Autodesk Inventor part; units mm, degrees
ref_plane "YZ Plane" through (0, 0, 0) normal (1, 0, 0) x (0, 1, 0)
ref_plane "XZ Plane" through (0, 0, 0) normal (0, 1, 0) x (-1, 0, 0)
ref_plane "XY Plane" through (0, 0, 0) normal (0, 0, 1) x (1, 0, 0)
sketch "Эскиз1" plane through (0, 0, 0) normal (1, 0, 0) x (0, 1, 0)
  circle A0 centre (0, 0) radius 30.5
  dimension "d0" = 61
extrude "Выдавливание1" add sketch "Эскиз1" along normal blind 25
sketch "Эскиз2" plane through (25, 0, 0) normal (1, 0, 0) x (0, 0, -1)
  circle A0 centre (0, 0) radius 41
  dimension "d3" = 82
extrude "Выдавливание2" add sketch "Эскиз2" along normal blind 26
sketch "Эскиз3" plane through (0, 0, 0) normal (0, 0, 1) x (1, 0, 0)
  line L0 (0, 0) -> (25, 0)
  line L1 (25, -30.5) -> (25, 30.5)
  circle A0 centre (12.5, 0) radius 3.5
  dimension "d6" = 7
extrude "Выдавливание3" cut sketch "Эскиз3" along normal through all both and the other way through all
sketch "Эскиз4" plane through (51, 0, 0) normal (1, 0, 0) x (0, 0, -1)
  circle A0 centre (0, 0) radius 30.5
  line L0 (0, 0) -> (-11.8974, 32.688)
  line L1 (0, 0) -> (0, 6.9467)
  circle A1 centre (-10.4316, 28.6606) radius 4
  line L2 (0, 0) -> (-31.5267, 14.7011)
  circle A2 centre (-27.6424, 12.8899) radius 4
  line L3 (0, 0) -> (-32.688, -11.8974)
  circle A3 centre (-28.6606, -10.4316) radius 4
  line L4 (0, 0) -> (-14.7011, -31.5267)
  circle A4 centre (-12.8899, -27.6424) radius 4
  line L5 (0, 0) -> (11.8974, -32.688)
  circle A5 centre (10.4316, -28.6606) radius 4
  line L6 (0, 0) -> (31.5267, -14.7011)
  circle A6 centre (27.6424, -12.8899) radius 4
  line L7 (0, 0) -> (32.688, 11.8974)
  circle A7 centre (28.6606, 10.4316) radius 4
  line L8 (0, 0) -> (14.7011, 31.5267)
  circle A8 centre (12.8899, 27.6424) radius 4
  dimension "d10" = 20
  dimension "d11" = 8
  dimension "d14" = 360
extrude "Выдавливание4" cut sketch "Эскиз4" against normal blind 10 contours A7 L7 A0 | A0 L7 A7 | A6 L6 A0 | A0 L6 A6 | L7 A7 A0 | A0 A7 L7 | L6 A6 A0 | A0 A6 L6 | A8 L8 A0 | A0 L8 A8 | A1 A0 L0 | L0 A0 A1 | A2 A0 L2 | L2 A0 A2 | A3 A0 L3 | L3 A0 A3 | A4 A0 L4 | L4 A0 A4 | A5 A0 L5 | L5 A0 A5 | A8 A0 L8 | A5 L5 A0 | A0 A8 L8 | L0 A1 A0 | A0 A1 L0 | L2 A2 A0 | A0 A2 L2 | L3 A3 A0 | A0 A3 L3 | L4 A4 A0 | A0 A4 L4 | L5 A5 A0
equation "\"Радиус_гибки\" = Толщина"
equation "\"Ширина_просечки\" = Толщина"
equation "\"Глубина_просечки\" = 0.5 * Толщина"
equation "\"Размер_просечки\" = 4 * Толщина"
equation "\"Мин_остаток\" = 2 * Толщина"
equation "\"Радиус_перехода\" = Радиус_гибки"
equation "\"Радиус_Якоби\" = Радиус_гибки"
equation "\"Размер_зазора\" = Толщина"
properties part number "хвостовик"
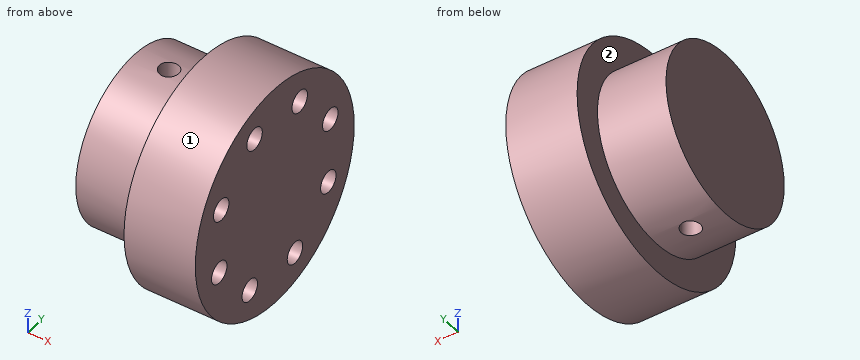
Could you check a few things on this model? Use its own coordinates, in mm. Face numbers are marked on the shaded views. A direction names the side the tool comes from. Coordinates: 2 decimals unless noted, no trailing zeros. Write each loop counter-clockwise with the first axis right and the second up, starting at its lowest first coordinate (ties: lowest second). Pieces come first, ordered by that corner, then holes. Notation, with made-up numbers: (-35.75, 83.25) -> (-7.75, 83.25) arc R36 cw to (-7.75, 119.25) -> close; hole circle Ø11 at (53, 70.25). An arc over 180 degrees is marked (long way). Return JSON: item names as keys, results as strings.
(1) Imagine slicing it at C-C, the plane x = 18. Please give me the cut outline in (y, z), then the cut area to 3 significant figures.
Numbers:
{"outline": "circle Ø61 at (0, 0)", "area": "2,920 mm2"}
(2) Imagine slicing it at D-D, the plane z = 12.5. Please give me the cut outline in (x, y), then the cut area to 3 significant figures.
Numbers:
{"outline": "(0, -27.82) -> (25, -27.82) -> (25, -39.05) -> (51, -39.05) -> (51, -31.62) -> (41, -31.62) -> (41, -23.66) -> (51, -23.66) -> (51, 25.24) -> (41, 25.24) -> (41, 32.08) -> (51, 32.08) -> (51, 39.05) -> (25, 39.05) -> (25, 27.82) -> (0, 27.82) -> close; hole circle Ø7 at (12.5, 0)", "area": "3,230 mm2"}
(3) I need wall thicknesses on L1, parallel to Y at x = 48, z = -13; L2, parallel to X at y = 34, z = -19. Which ranges of each line are inside material? Lowest first, please.
Numbers:
{"L1": "y = -38.88 to -31.73, -25.59 to 23.64, 31.64 to 38.88", "L2": "x = 25 to 51"}
(4) Imagine slicing it at B-B, the plane z = 0. Please give me the cut outline in (x, y).
Numbers:
{"outline": "(0, -30.5) -> (25, -30.5) -> (25, -41) -> (51, -41) -> (51, 41) -> (25, 41) -> (25, 30.5) -> (0, 30.5) -> close; hole circle Ø7 at (12.5, 0)"}
(5) Imagine slicing it at A-A, the plane y = 0. Please give me the cut outline in (x, z), then the cut area to 3 significant figures.
Numbers:
{"outline": "(0, -30.5) -> (9, -30.5) -> (9, 30.5) -> (0, 30.5) -> close; (16, -30.5) -> (25, -30.5) -> (25, -41) -> (51, -41) -> (51, 41) -> (25, 41) -> (25, 30.5) -> (16, 30.5) -> close", "area": "3,230 mm2"}
(6) Which directions (+Z, -Z, +X, -X, +Y, -Y) give clear straight access to the entire face, cutting with the end or side of a thin tool? Please do the marked faces 1 and 2.
Numbers:
{"face 1": "+X, -X", "face 2": "-X"}
(7) I'm going to push flat-ended pins straight in: pin 1 (2 mm diameter, centred on x = 21.5, y = -16, fed in from +Z); pin 2 (2.5 mm diameter, centred on y = -9, z = 28.5, fed in from +X); pin 3 (6 mm diameter, centred on x = 11, z = -18.5, fed in from +Y). Where does each tip first touch, or does it pass through?
Numbers:
{"pin 1": "stops at z = 26.56", "pin 2": "stops at x = 41", "pin 3": "stops at y = 26.27"}
